Read the model definition and answer for the solid it produces. Units are mm, in the model's axes. A direction names the side the tool comes from. Coordinates: 2 decimals unless noted, no trailing zeros. Write each loop counter-clockwise with the first axis right and the second up, starting at its lowest first coordinate (ties: lowest second). Pieces come first, ordered by that corner, then holes. Notation, with made-up numbers: M 9,18 L 47,18 A5 ccw 47,23 Z; hole C -3.75,70 d2. An arc over 180 degrees is marked long. Use a Markdown table: item, result. Add a question column.
from build123d import *

# Parameters (mm, degrees)
LOFTED_BENDS1_DEPTH = 100
SKETCH11_R          = 2.5
CUT_EXTRUDE1_DEPTH  = 137.408236331


# Read off the part's stored shape, not the designer's step: Lofted Bends1
with BuildPart() as part:
    # Lofted Bends1 outline → Lofted Bends1 (new body)
    with BuildSketch(Plane.XY):
        with BuildLine():
            Line((20.207259422, 35), (20.207259422, 37))
            Line((20.207259422, 37), (-19.781983213, 37))
            ThreePointArc((-19.781983213, 37), (-21.150283213, 36.63336512), (-22.151948333, 35.6317))
            Line((-22.151948333, 35.6317), (-41.933931547, 1.3683))
            ThreePointArc((-41.933931547, 1.3683), (-42.300566427, 0), (-41.933931547, -1.3683))
            Line((-41.933931547, -1.3683), (-22.151948333, -35.6317))
            ThreePointArc((-22.151948333, -35.6317), (-21.150283213, -36.63336512), (-19.781983213, -37))
            Line((-19.781983213, -37), (19.781983213, -37))
            ThreePointArc((19.781983213, -37), (21.150283213, -36.63336512), (22.151948333, -35.6317))
            Line((22.151948333, -35.6317), (41.933931547, -1.3683))
            ThreePointArc((41.933931547, -1.3683), (42.300566427, 0), (41.933931547, 1.3683))
            Line((41.933931547, 1.3683), (22.514616839, 35.003539722))
            Line((22.514616839, 35.003539722), (20.782566032, 34.003539722))
            Line((20.782566032, 34.003539722), (40.201880739, 0.3683))
            ThreePointArc((40.201880739, 0.3683), (40.300566427, 0), (40.201880739, -0.3683))
            Line((40.201880739, -0.3683), (20.419897526, -34.6317))
            ThreePointArc((20.419897526, -34.6317), (20.150283213, -34.901314312), (19.781983213, -35))
            Line((19.781983213, -35), (-19.781983213, -35))
            ThreePointArc((-19.781983213, -35), (-20.150283213, -34.901314312), (-20.419897526, -34.6317))
            Line((-20.419897526, -34.6317), (-40.201880739, -0.3683))
            ThreePointArc((-40.201880739, -0.3683), (-40.300566427, 0), (-40.201880739, 0.3683))
            Line((-40.201880739, 0.3683), (-20.419897526, 34.6317))
            ThreePointArc((-20.419897526, 34.6317), (-20.150283213, 34.901314312), (-19.781983213, 35))
            Line((-19.781983213, 35), (20.207259422, 35))
        make_face()
    extrude(amount=LOFTED_BENDS1_DEPTH)

    # Sketch11 → Cut-Extrude1 (cut, through all)
    with BuildSketch(Plane(origin=(32.04293994, 18.5, 0), x_dir=(0, 0, -1), z_dir=(0.8660254037844385, 0.5000000000000004, 0))):
        with Locations(Location((-89.390171196, -0.362668506, 0), (0, 0, 270))):
            Circle(SKETCH11_R)
    extrude(amount=-CUT_EXTRUDE1_DEPTH, mode=Mode.SUBTRACT)


solid = part.part
Item 1: Consider probe 1 along X at (y, z) = (0, 11.5); probe 2 along Y at (x, z) = (-12, 30); probe 3 along Y at (x, z) = (33, 13). Determine where each line is inside the solid, lowest interval first.
Item 2: For faces 1 (the cylindrical face through (21.133, -36.643, 49.3)), 2 (the flat face through (-30.172, -17.74, 49.3)), determine the directions among +Z, -Z, +X, -X, +Y, -Y from which every point of the face is accessible in a straight line to the end or side of a thin tool.
Item 3: Find section A-A on x = 2. Give the vertices of the cut face in (y, z), then the cut area to 3 significant figures.
Item 4: Find section C-C on z = 70. Give the vertices of the cut face in (x, y), then the cut area to 3 significant figures.
Item 5: Determine the mould class of faces 3 (the flat face through (-0.2, -35.5, 100)), 4 (the cylindrical face through (-31.15, -18.03, 86.91)), 5 (the flat face through (-0.2, -35.5, 0)), 6 (the flat face through (30.356, 17.421, 49.3)) for opening direction Z: pulls with the +Z half, pulls with the -Z half, needs draft (parallel to the pull), parting line crosses it, or undercut.
Item 6: Find section B-B on y = -11.5. Give the vertices of the cut face in (x, z) (3 decimals), then the cut area to 3 significant figures.
Item 7: Each of these flat-tipped pins is pushed along its axis until it touches: pin 1 (12 mm diameter, centred on y = 11, z = 48.5, fed in from +X); pin 2 (6 mm diameter, centred on y = -26.5, z = 34, fed in from -X); pin 3 (1 mm diameter, centred on x = -32, z = 37.5, fed in from -Y). Where does it stop, or does it pass through?
Geometry says:
| question | item | result |
|---|---|---|
| 1 | probe 1 | x = -42.3 to -40.3, 40.3 to 42.3 |
| 1 | probe 2 | y = -37 to -35, 35 to 37 |
| 1 | probe 3 | y = -16.84 to -12.84, 12.84 to 16.84 |
| 2 | face 1 | +Z, -Z, +X, -Y |
| 2 | face 2 | +Z, -Z |
| 3 | outline | M -37,0 L -35,0 L -35,100 L -37,100 Z; M 35,0 L 37,0 L 37,100 L 35,100 Z |
| 3 | area | 400 mm2 |
| 4 | outline | M -41.93,-1.37 L -22.15,-35.63 A2.74 ccw -19.78,-37 L 19.78,-37 A2.74 ccw 22.15,-35.63 L 41.93,-1.37 A2.74 ccw 41.93,1.37 L 22.51,35 L 20.78,34 L 40.2,0.37 A0.74 cw 40.2,-0.37 L 20.42,-34.63 A0.74 cw 19.78,-35 L -19.78,-35 A0.74 cw -20.42,-34.63 L -40.2,-0.37 A0.74 cw -40.2,0.37 L -20.42,34.63 A0.74 cw -19.78,35 L 20.21,35 L 20.21,37 L -19.78,37 A2.74 ccw -22.15,35.63 L -41.93,1.37 A2.74 ccw Z |
| 4 | area | 492 mm2 |
| 5 | face 3 | pulls with the +Z half |
| 5 | face 4 | undercut |
| 5 | face 5 | pulls with the -Z half |
| 5 | face 6 | needs draft |
| 6 | outline | M -36.084,0 L -33.775,0 L -33.775,100 L -36.084,100 Z; M 33.775,0 L 36.084,0 L 36.084,100 L 33.775,100 Z |
| 6 | area | 462 mm2 |
| 7 | pin 1 | stops at x = 39.84 |
| 7 | pin 2 | stops at x = -29.16 |
| 7 | pin 3 | stops at y = -19.44 |
